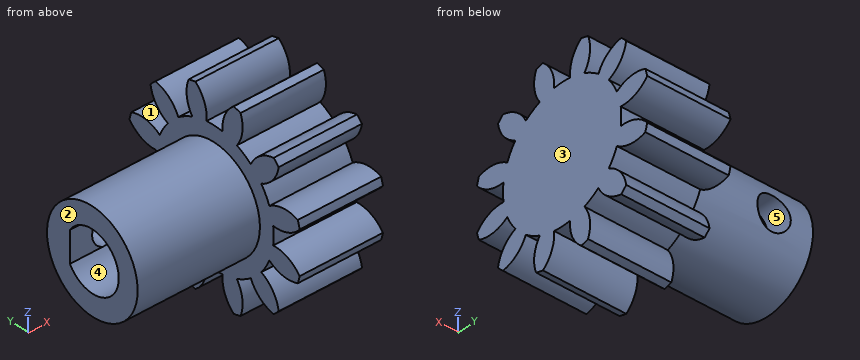
```python
from build123d import *

# Parameters (mm, degrees)
BASPROSKE_W         = 9.525
BASPROSKE_H         = 11.1125
TOOTHCUT_DEPTH      = 19.376641083
TEETHCUTS_COUNT     = 12
BORSKE_R            = 3.175
BORE_DEPTH          = 9.525
BOSS_EXTRUDE1_START = -25.4
SKETCH2_R           = 7.539355
BOSS_EXTRUDE1_DEPTH = 25.4
CUT_EXTRUDE1_DEPTH  = 23.495
SKETCH5_R           = 1.905
CUT_EXTRUDE2_DEPTH  = 24.605363577
SKETCH6_R           = 12.7
SKETCH6_R_2         = 5.7785
CUT_EXTRUDE3_DEPTH  = 15.875
SKETCH7_R           = 5.7785
CUT_EXTRUDE5_DEPTH  = 1.905
FILLET1_R           = 1.058333333


with BuildPart() as part:
    # BasProSke → Base-Revolve (revolve)
    with BuildSketch(Plane(origin=(0, 0, 0), x_dir=(1, 0, 0), z_dir=(0, 1, 0)), mode=Mode.PRIVATE) as base_revolve_sk:
        with Locations((4.7625, 5.55625)):
            Rectangle(BASPROSKE_W, BASPROSKE_H)
    revolve(base_revolve_sk.sketch.rotate(Axis((-10, 0, 0), (1, 0, 0)), 180), axis=Axis((-10, 0, 0), (1, 0, 0)))

    # TooCutSke → ToothCut (cut, through all)
    with BuildSketch(Plane(origin=(0, 0, 0), x_dir=(0, 0, -1), z_dir=(1, 0, 0))):
        with BuildLine():
            ThreePointArc((1.026937745, 7.469087808), (0, 7.539355), (-1.026937745, 7.469087808))
            ThreePointArc((-1.026937745, 7.469087808), (-1.30857978, 9.35080814), (-2.465050847, 10.861691431))
            ThreePointArc((-2.465050847, 10.861691431), (0, 11.1379), (2.465050847, 10.861691431))
            ThreePointArc((2.465050847, 10.861691431), (1.30857978, 9.35080814), (1.026937745, 7.469087808))
        make_face()
    toothcut = extrude(amount=TOOTHCUT_DEPTH, mode=Mode.SUBTRACT)

    # TeethCuts: ToothCut ×12 about axis
    teethcuts_axis = Axis((0, 0, 0), (1, 0, 0))
    for i in range(1, TEETHCUTS_COUNT):
        add(toothcut.rotate(teethcuts_axis, i * 360 / TEETHCUTS_COUNT), mode=Mode.SUBTRACT)

    # BorSke → Bore (cut, symmetric)
    with BuildSketch(Plane(origin=(0, 0, 0), x_dir=(0, 0, -1), z_dir=(1, 0, 0))):
        with Locations(Location((0, 0, 0), (0, 0, 180))):
            Circle(BORSKE_R)
    extrude(amount=BORE_DEPTH, both=True, mode=Mode.SUBTRACT)

    # Sketch2 → Boss-Extrude1 (add)
    with BuildSketch(Plane(origin=(9.525, 0, 0), x_dir=(0, 0, -1), z_dir=(1, 0, 0)).offset(BOSS_EXTRUDE1_START)):
        with Locations(Location((0, 0, 0), (0, 0, 172.171388978))):
            Circle(SKETCH2_R)
    extrude(amount=BOSS_EXTRUDE1_DEPTH)

    # Sketch3 → Cut-Extrude1 (cut)
    with BuildSketch(Plane.ZY.offset(15.875)):
        with BuildLine():
            Line((-1.778, 2.8575), (1.778, 2.8575))
            ThreePointArc((1.778, 2.8575), (0, -3.3655), (-1.778, 2.8575))
        make_face()
    extrude(amount=-CUT_EXTRUDE1_DEPTH, mode=Mode.SUBTRACT)

    # Sketch5 → Cut-Extrude2 (cut, through all)
    with BuildSketch(Plane.XZ.offset(-2.8575)):
        with Locations(Location((-9.525, 0, 0), (0, 0, 270))):
            Circle(SKETCH5_R)
    extrude(amount=-CUT_EXTRUDE2_DEPTH, mode=Mode.SUBTRACT)

    # Sketch6 → Cut-Extrude3 (cut)
    with BuildSketch(Plane.ZY.offset(15.875)):
        Circle(SKETCH6_R)
        Circle(SKETCH6_R_2, mode=Mode.SUBTRACT)
    extrude(amount=-CUT_EXTRUDE3_DEPTH, mode=Mode.SUBTRACT)

    # Sketch7 → Cut-Extrude5 (cut)
    with BuildSketch(Plane.ZY.offset(15.875)):
        Circle(SKETCH7_R)
    extrude(amount=-CUT_EXTRUDE5_DEPTH, mode=Mode.SUBTRACT)

    # Fillet1
    # the kernel refuses this fillet: 1.058333333 mm, written as the material it adds along each edge
    with BuildSketch(Plane(origin=(7.62, 0, 0), x_dir=(0, 0.9999950652018581, 0.0031415874858805883), z_dir=(0, 0.0031415874858805883, -0.9999950652018581))) as fillet1_piece_1:
        with BuildLine():
            CenterArc((3.3655 - FILLET1_R, -FILLET1_R), FILLET1_R, 0, 90)
            Line((3.3655 - FILLET1_R, 0), (3.3655, 0))
            Line((3.3655, 0), (3.3655, -FILLET1_R))
        make_face()
    revolve(axis=Axis((7.62, 0, 0), (1, 0, 0)), revolution_arc=359.64)
    with BuildSketch(Plane(origin=(7.62, 2.8575, -4.423833333), x_dir=(-1, 0, 0), z_dir=(0, 0, 1))) as fillet1_piece_2:
        with BuildLine():
            CenterArc((FILLET1_R, FILLET1_R), FILLET1_R, 180, 90)
            Line((0, FILLET1_R), (0, 0))
            Line((0, 0), (FILLET1_R, 0))
        make_face()
    extrude(amount=8.847666667)


solid = part.part
```
For this review, take the finished solid that the model builds, in its own axes (mm). Face numbers are marked on the shaded views. A direction names the side the tool comes from. Coordinates: 2 decimals unless noted, no trailing zeros. Order: outer loops, then holes, each group sorted by start corner. A loop starts at its lowest first (then second) coordinate and runs counter-clockwise, first axis right, second up. Notation, with made-up numbers: (-8.75, 56.5) - (-0.75, 56.5) arc R22 cw to (-0.75, 78.5) - close; hole circle Ø11 at (86.5, 76). An arc over 180 degrees is marked (long way). Answer as a JSON object with one key per item and string values. Group by question number.
1. We need section B-B on x = -1.5. State the section outline as (y, z) points.
2. We need section A-A on z = 0. State the section outline as (x, y) points (1 decimal), then the cut area to 3 significant figures.
3. For probe 1 along X at (y, z) = (3, -8.5) (3 decimals); probe 2 along Z at (x, y) = (1, -1.5); probe 3 along X at (y, z) = (3.65, 0) (3 decimals), list the stretches that pass through material, from the lowest coordinate up.
4. Clearance check with flat-ended pins moving along their axes: P1, Ø3, axis at x = -11, y = -1, coming from the +Z side; P2, Ø6, axis at x = -9.525, z = 0, coming from the -Y side; P3, Ø10, axis at x = 4.5, y = 0, coming from the +Z side; P4, Ø1.5, axis at x = -1, y = -8.5, coming from the -Z side. State where each tip first meets the part, or that it passes through.
5. We need section D-D on y = 8.75. State the section outline as (x, z) points (3 decimals).
6. For the marked faces 3, 4 and 5, list the 3-axis set-ups (+Z, -Z, +X, -X, +Y, -Y) from which the entire face can be reached by the end or side of a thin tool; tool diameter is ignored.
7. The part is to be moulded in two halves that separate along Y. For the marked faces 1 and 2, say which applies: pulls with the +Y half, pulls with the -Y half, needs draft (parallel to the pull), parting line crosses it, or undercut.
8. We need section C-C on y = 0. State the section outline as (x, z) points (1 decimal), then the cut area to 3 significant figures.
Final values:
{
 "1": {"outline": "circle Ø11.56 at (0, 0); hole (2.86, -1.78) - (2.86, 1.78) arc R3.37 ccw (long way) to start"},
 "2": {"outline": "(-14, -5.8) - (0, -5.8) - (0, -7.5) - (9.5, -7.5) - (9.5, 7.5) - (0, 7.5) - (0, 5.8) - (-7.6, 5.8) - (-7.6, 2.9) - (6.6, 2.9) arc R1.1 cw to (7.6, 1.8) - (7.6, -2.3) arc R1.1 cw to (6.6, -3.4) - (-14, -3.4) - close; (-14, 2.9) - (-11.4, 2.9) - (-11.4, 5.8) - (-14, 5.8) - close", "area": "160 mm²"},
 "3": {"probe 1": "0 to 9.525", "probe 2": "-9.74 to -3.01, 3.01 to 9.74", "probe 3": "-13.97 to -11.43, -7.62 to 9.525"},
 "4": {"P1": "z = 5.78", "P2": "y = -5.78", "P3": "z = 10.84", "P4": "through"},
 "5": {"outline": "(0, -3.542) - (9.525, -3.542) - (9.525, -1.111) - (0, -1.111) - close; (0, 1.111) - (9.525, 1.111) - (9.525, 3.542) - (0, 3.542) - close"},
 "6": {"face 3": "+Z, -Z, +X, +Y, -Y", "face 4": "-X", "face 5": "+Y"},
 "7": {"face 1": "undercut", "face 2": "needs draft"},
 "8": {"outline": "(-14, -5.8) - (0, -5.8) - (0, -7.5) - (9.5, -7.5) - (9.5, 7.5) - (0, 7.5) - (0, 5.8) - (-14, 5.8) - (-14, 3.4) - (6.6, 3.4) arc R1.1 cw to (7.6, 2.3) - (7.6, -2.3) arc R1.1 cw to (6.6, -3.4) - (-14, -3.4) - close", "area": "160 mm²"}
}
